Check sheet for the modelled part. Datum: model origin and axes. Units: mm. A direction names the side the tool comes from. Give positions to 0.01 mm unless a question says otherwise; leave off trailing zeros. Order: outer loops, then holes, each group sorted by start corner. A loop starts at its lowest first (then second) coordinate and runs counter-clockwise, first axis right, second up. Notation, with made-up numbers: M 10.5,-15 L 16.5,-15 A15 cw 16.5,-9 Z; hole C 14,36 d11. An arc over 180 degrees is marked long. One line per question, with ' | ' between items. Start each with the question number.
```python
from build123d import *

# Parameters (mm, degrees)
SKETCH_1_W           = 10
SKETCH_1_H           = 10
SKETCH_1_W_2         = 6.2
SKETCH_1_H_2         = 6.2
EXTRUDE_1_DEPTH      = 4
SKETCH_1_R           = 1.25
EXTRUDE_1_2_DEPTH    = 4
EXTRUDE_START        = 4
SKETCH_1_3_W         = 10
SKETCH_1_3_H         = 10
EXTRUDE_2_DEPTH      = 1
SKETCH_2_W           = 7.8
SKETCH_2_H           = 7.8
EXTRUDE_3_DEPTH      = 10
SKETCH_3_R           = 2.5
CUT_EXTRUDE_1_DEPTH  = 19.144145061
SKETCH_3_3_R         = 3.15
SKETCH_3_3_R_2       = 2.5
CUT_EXTRUDE_2_DEPTH  = 1.5
CUT_EXTRUDE_START    = -6.3
SKETCH_3_4_R         = 3.15
SKETCH_3_4_R_2       = 2.5
CUT_EXTRUDE_3_DEPTH  = 1.5
SKETCH_4_R           = 1
SKETCH_4_R_2         = 0.7
CUT_EXTRUDE_4_DEPTH  = 1
CUT_EXTRUDE_START_2  = -9
SKETCH_4_2_R         = 1
SKETCH_4_2_R_2       = 0.7
CUT_EXTRUDE_5_DEPTH  = 1
CUT_EXTRUDE_6_REACH  = 20.708
SKETCH_4_3_R         = 0.7
CUT_EXTRUDE_START_3  = -10
SKETCH_4_4_R         = 0.7
CUT_EXTRUDE_7_DEPTH  = 1.9
CUT_EXTRUDE_8_REACH  = 20.708
SKETCH_5_R           = 0.7
SKETCH_5_3_R         = 0.7
CUT_EXTRUDE_9_DEPTH  = 1.9
SKETCH_5_4_R         = 1
CUT_EXTRUDE_10_DEPTH = 1
SKETCH_5_5_R         = 1
CUT_EXTRUDE_11_DEPTH = 1


with BuildPart() as part:
    # Sketch 1 → Extrude 1 (new body)
    with BuildSketch(Plane(origin=(0, 0, 0), x_dir=(1, 0, 0), z_dir=(0, 1, 0))):
        Rectangle(SKETCH_1_W, SKETCH_1_H)
        Rectangle(SKETCH_1_W_2, SKETCH_1_H_2, mode=Mode.SUBTRACT)
    extrude(amount=EXTRUDE_1_DEPTH)



with BuildPart() as body_2:
    # Sketch 1 → Extrude 1 2 (new body)
    with BuildSketch(Plane(origin=(0, 0, 0), x_dir=(1, 0, 0), z_dir=(0, 1, 0))):
        with Locations(Location((0, 0, 0), (0, 0, 270))):
            Circle(SKETCH_1_R)
    extrude(amount=EXTRUDE_1_2_DEPTH)


with BuildPart() as part_1:
    add(part.part)

    add(body_2.part)  # Extrude 2 merges body 2
    # Sketch 1_3 → Extrude 2 (add)
    with BuildSketch(Plane(origin=(0, 0, 0), x_dir=(1, 0, 0), z_dir=(0, 1, 0)).offset(EXTRUDE_START)):
        Rectangle(SKETCH_1_3_W, SKETCH_1_3_H)
    extrude(amount=EXTRUDE_2_DEPTH)

    # Sketch 2 → Extrude 3 (add)
    with BuildSketch(Plane(origin=(0, 5, 0), x_dir=(1, 0, 0), z_dir=(0, 1, 0))):
        Rectangle(SKETCH_2_W, SKETCH_2_H)
    extrude(amount=EXTRUDE_3_DEPTH)

    # Sketch 3 → Cut-Extrude 1 (cut, through all)
    with BuildSketch(Plane(origin=(3.9, 0, 0), x_dir=(0, 0, -1), z_dir=(1, 0, 0))):
        with Locations((0, 11.1)):
            Circle(SKETCH_3_R)
    extrude(amount=-CUT_EXTRUDE_1_DEPTH, mode=Mode.SUBTRACT)

    # Sketch 3_3 → Cut-Extrude 2 (cut)
    with BuildSketch(Plane(origin=(3.9, 0, 0), x_dir=(0, 0, -1), z_dir=(1, 0, 0))):
        with Locations((0, 11.1)):
            Circle(SKETCH_3_3_R)
        with Locations((0, 11.1)):
            Circle(SKETCH_3_3_R_2, mode=Mode.SUBTRACT)
    extrude(amount=-CUT_EXTRUDE_2_DEPTH, mode=Mode.SUBTRACT)

    # Sketch 3_4 → Cut-Extrude 3 (cut)
    with BuildSketch(Plane(origin=(3.9, 0, 0), x_dir=(0, 0, -1), z_dir=(1, 0, 0)).offset(CUT_EXTRUDE_START)):
        with Locations((0, 11.1)):
            Circle(SKETCH_3_4_R)
        with Locations((0, 11.1)):
            Circle(SKETCH_3_4_R_2, mode=Mode.SUBTRACT)
    extrude(amount=-CUT_EXTRUDE_3_DEPTH, mode=Mode.SUBTRACT)

    # Sketch 4 → Cut-Extrude 4 (cut)
    with BuildSketch(Plane(origin=(5, 0, 0), x_dir=(0, 0, -1), z_dir=(1, 0, 0))):
        with Locations((0, 2.5)):
            Circle(SKETCH_4_R)
        with Locations((0, 2.5)):
            Circle(SKETCH_4_R_2, mode=Mode.SUBTRACT)
    extrude(amount=-CUT_EXTRUDE_4_DEPTH, mode=Mode.SUBTRACT)

    # Sketch 4_2 → Cut-Extrude 5 (cut)
    with BuildSketch(Plane(origin=(5, 0, 0), x_dir=(0, 0, -1), z_dir=(1, 0, 0)).offset(CUT_EXTRUDE_START_2)):
        with Locations((0, 2.5)):
            Circle(SKETCH_4_2_R)
        with Locations((0, 2.5)):
            Circle(SKETCH_4_2_R_2, mode=Mode.SUBTRACT)
    extrude(amount=-CUT_EXTRUDE_5_DEPTH, mode=Mode.SUBTRACT)

    # Sketch 4_3 → Cut-Extrude 6 (cut, up to next)
    with BuildSketch(Plane(origin=(5, 0, 0), x_dir=(0, 0, -1), z_dir=(1, 0, 0)), mode=Mode.PRIVATE) as cut_extrude_6_sk1:
        with Locations(Location((0, 2.5, 0), (0, 0, 180))):
            Circle(SKETCH_4_3_R)
    cut_extrude_6_tool1 = extrude(cut_extrude_6_sk1.sketch, amount=-CUT_EXTRUDE_6_REACH, mode=Mode.PRIVATE) & part_1.part
    add(cut_extrude_6_tool1.solids().sort_by_distance((5, 2.5, 0))[0], mode=Mode.SUBTRACT)

    # Sketch 4_4 → Cut-Extrude 7 (cut)
    with BuildSketch(Plane(origin=(5, 0, 0), x_dir=(0, 0, -1), z_dir=(1, 0, 0)).offset(CUT_EXTRUDE_START_3)):
        with Locations((0, 2.5)):
            Circle(SKETCH_4_4_R)
    extrude(amount=CUT_EXTRUDE_7_DEPTH, mode=Mode.SUBTRACT)

    # Sketch 5 → Cut-Extrude 8 (cut, up to next)
    with BuildSketch(Plane(origin=(0, 0, -5), x_dir=(-1, 0, 0), z_dir=(0, 0, -1)), mode=Mode.PRIVATE) as cut_extrude_8_sk1:
        with Locations((0, 2.5)):
            Circle(SKETCH_5_R)
    cut_extrude_8_tool1 = extrude(cut_extrude_8_sk1.sketch, amount=-CUT_EXTRUDE_8_REACH, mode=Mode.PRIVATE) & part_1.part
    add(cut_extrude_8_tool1.solids().sort_by_distance((0, 2.5, -5))[0], mode=Mode.SUBTRACT)

    # Sketch 5_3 → Cut-Extrude 9 (cut)
    with BuildSketch(Plane(origin=(0, 0, -5), x_dir=(-1, 0, 0), z_dir=(0, 0, -1)).offset(CUT_EXTRUDE_START_3)):
        with Locations((0, 2.5)):
            Circle(SKETCH_5_3_R)
    extrude(amount=CUT_EXTRUDE_9_DEPTH, mode=Mode.SUBTRACT)

    # Sketch 5_4 → Cut-Extrude 10 (cut)
    with BuildSketch(Plane(origin=(0, 0, -5), x_dir=(-1, 0, 0), z_dir=(0, 0, -1))):
        with Locations((0, 2.5)):
            Circle(SKETCH_5_4_R)
    extrude(amount=-CUT_EXTRUDE_10_DEPTH, mode=Mode.SUBTRACT)

    # Sketch 5_5 → Cut-Extrude 11 (cut)
    with BuildSketch(Plane(origin=(0, 0, -5), x_dir=(-1, 0, 0), z_dir=(0, 0, -1)).offset(CUT_EXTRUDE_START_2)):
        with Locations((0, 2.5)):
            Circle(SKETCH_5_5_R)
    extrude(amount=-CUT_EXTRUDE_11_DEPTH, mode=Mode.SUBTRACT)


solid = part_1.part
```
Item 1: Draft check along Z on faces 4 (the face through (3.9, 7.7, 0.1)), 5 (the face through (0, 1, -5)), 6 (the face through (3.16, 8.025, 0.683)). Enter one of: released by +Z, released by -Z, zero draft, split by the parting line, or undercut.
Item 2: Go/stop test with flat-tipped pins: P1, Ø4, axis at x = -3, y = 10, coming from the +Z side; P2, Ø1.2, axis at y = 2.5, z = 0, coming from the -X side; P3, Ø0.8, axis at x = 0, y = 2.5, coming from the +Z side. Record where each tip stops, or that it passes through.
Item 3: Scan lines: probe 1 along X at (y, z) = (2, 2.25); probe 2 along Y at (x, z) = (-0.2, 0); probe 3 along Y at (x, z) = (-2.85, 0). Record each from-to range of solid material in increasing order. Write a range as [from, to].
Item 4: Section check A-A, the plane x = 0. State how many separate pieces and enclosed holes the cut face has, then the cut area to 3 significant figures.
Item 5: Section check B-B, the plane y = 11.1. Record the cut outline in (x, z).
Item 6: Set-up check for faces 1 (the face through (-3.56, 2.97, 0.52)), 2 (the face through (0, 1.5, -3.1)), 3 (the face through (0.52, 2.97, 3.56)): record each of +Z, -Z, +X, -X, +Y, -Y from which the full face is reachable in a straight line by a thin tool's end or side.
Item 7: Section check C-C, the plane x = -4.25. Record the cut outline in (y, z).
Reported:
1) face 4: zero draft | face 5: released by -Z | face 6: undercut
2) P1: stops at z = 3.9 | P2: stops at x = -1.25 | P3: stops at z = 1.25
3) probe 1: x = [-5, -3.1], [3.1, 5] | probe 2: y = [0, 8.6], [13.6, 15] | probe 3: y = [4, 7.95], [14.25, 15]
4) separate pieces: 3 | enclosed holes: 1 | area: 87.0 mm^2
5) outline: M -3.9,-3.9 L 3.9,-3.9 L 3.9,-3.15 L 2.4,-3.15 L 2.4,-2.5 L -2.4,-2.5 L -2.4,-3.15 L -3.9,-3.15 Z; M -3.9,3.15 L -2.4,3.15 L -2.4,2.5 L 2.4,2.5 L 2.4,3.15 L 3.9,3.15 L 3.9,3.9 L -3.9,3.9 Z
6) face 1: -X | face 2: -Y | face 3: +Z
7) outline: M 0,-5 L 5,-5 L 5,5 L 0,5 Z; hole C 2.5,0 d2
